```python
from build123d import *

# Parameters (mm, degrees)
SKETCH1_R           = 1.85
SKETCH1_R_2         = 4
BOSS_EXTRUDE1_DEPTH = 2


with BuildPart() as part:
    # Sketch1 → Boss-Extrude1 (new body)
    with BuildSketch(Plane.XZ):
        with BuildLine():
            Line((48, -174), (48, 14))
            ThreePointArc((48, 14), (47.414213562, 15.414213562), (46, 16))
            Line((46, 16), (-14, 16))
            ThreePointArc((-14, 16), (-15.414213562, 15.414213562), (-16, 14))
            Line((-16, 14), (-16, -174))
            ThreePointArc((-16, -174), (-15.414213562, -175.414213562), (-14, -176))
            Line((-14, -176), (46, -176))
            ThreePointArc((46, -176), (47.414213562, -175.414213562), (48, -174))
        make_face()
        with Locations((37.656854249, -154.343145751)):
            Circle(SKETCH1_R, mode=Mode.SUBTRACT)
        with Locations((26.343145751, -154.343145751)):
            Circle(SKETCH1_R, mode=Mode.SUBTRACT)
        with Locations((26.343145751, -165.656854249)):
            Circle(SKETCH1_R, mode=Mode.SUBTRACT)
        with Locations((37.656854249, -165.656854249)):
            Circle(SKETCH1_R, mode=Mode.SUBTRACT)
        with Locations((24, -160)):
            Circle(SKETCH1_R, mode=Mode.SUBTRACT)
        with Locations((32, -152)):
            Circle(SKETCH1_R, mode=Mode.SUBTRACT)
        with Locations((40, -160)):
            Circle(SKETCH1_R, mode=Mode.SUBTRACT)
        with Locations((32, -168)):
            Circle(SKETCH1_R, mode=Mode.SUBTRACT)
        with Locations((32, -160)):
            Circle(SKETCH1_R_2, mode=Mode.SUBTRACT)
        with Locations((5.656854249, -154.343145751)):
            Circle(SKETCH1_R, mode=Mode.SUBTRACT)
        with Locations((-5.656854249, -154.343145751)):
            Circle(SKETCH1_R, mode=Mode.SUBTRACT)
        with Locations((-5.656854249, -165.656854249)):
            Circle(SKETCH1_R, mode=Mode.SUBTRACT)
        with Locations((5.656854249, -165.656854249)):
            Circle(SKETCH1_R, mode=Mode.SUBTRACT)
        with Locations((-8, -160)):
            Circle(SKETCH1_R, mode=Mode.SUBTRACT)
        with Locations((0, -152)):
            Circle(SKETCH1_R, mode=Mode.SUBTRACT)
        with Locations((8, -160)):
            Circle(SKETCH1_R, mode=Mode.SUBTRACT)
        with Locations((0, -168)):
            Circle(SKETCH1_R, mode=Mode.SUBTRACT)
        with Locations((0, -160)):
            Circle(SKETCH1_R_2, mode=Mode.SUBTRACT)
        with Locations((37.656854249, -122.34314575)):
            Circle(SKETCH1_R, mode=Mode.SUBTRACT)
        with Locations((26.343145751, -122.34314575)):
            Circle(SKETCH1_R, mode=Mode.SUBTRACT)
        with Locations((26.343145751, -133.656854249)):
            Circle(SKETCH1_R, mode=Mode.SUBTRACT)
        with Locations((37.656854249, -133.656854249)):
            Circle(SKETCH1_R, mode=Mode.SUBTRACT)
        with Locations((24, -128)):
            Circle(SKETCH1_R, mode=Mode.SUBTRACT)
        with Locations((32, -120)):
            Circle(SKETCH1_R, mode=Mode.SUBTRACT)
        with Locations((40, -128)):
            Circle(SKETCH1_R, mode=Mode.SUBTRACT)
        with Locations((32, -136)):
            Circle(SKETCH1_R, mode=Mode.SUBTRACT)
        with Locations((32, -128)):
            Circle(SKETCH1_R_2, mode=Mode.SUBTRACT)
        with Locations((5.656854249, -122.34314575)):
            Circle(SKETCH1_R, mode=Mode.SUBTRACT)
        with Locations((-5.656854249, -122.34314575)):
            Circle(SKETCH1_R, mode=Mode.SUBTRACT)
        with Locations((-5.656854249, -133.656854249)):
            Circle(SKETCH1_R, mode=Mode.SUBTRACT)
        with Locations((5.656854249, -133.656854249)):
            Circle(SKETCH1_R, mode=Mode.SUBTRACT)
        with Locations((-8, -128)):
            Circle(SKETCH1_R, mode=Mode.SUBTRACT)
        with Locations((0, -120)):
            Circle(SKETCH1_R, mode=Mode.SUBTRACT)
        with Locations((8, -128)):
            Circle(SKETCH1_R, mode=Mode.SUBTRACT)
        with Locations((0, -136)):
            Circle(SKETCH1_R, mode=Mode.SUBTRACT)
        with Locations((0, -128)):
            Circle(SKETCH1_R_2, mode=Mode.SUBTRACT)
        with Locations((37.656854249, -90.343145751)):
            Circle(SKETCH1_R, mode=Mode.SUBTRACT)
        with Locations((26.343145751, -90.343145751)):
            Circle(SKETCH1_R, mode=Mode.SUBTRACT)
        with Locations((26.343145751, -101.65685425)):
            Circle(SKETCH1_R, mode=Mode.SUBTRACT)
        with Locations((37.656854249, -101.65685425)):
            Circle(SKETCH1_R, mode=Mode.SUBTRACT)
        with Locations((24, -96)):
            Circle(SKETCH1_R, mode=Mode.SUBTRACT)
        with Locations((32, -88)):
            Circle(SKETCH1_R, mode=Mode.SUBTRACT)
        with Locations((40, -96)):
            Circle(SKETCH1_R, mode=Mode.SUBTRACT)
        with Locations((32, -104)):
            Circle(SKETCH1_R, mode=Mode.SUBTRACT)
        with Locations((32, -96)):
            Circle(SKETCH1_R_2, mode=Mode.SUBTRACT)
        with Locations((5.656854249, -90.343145751)):
            Circle(SKETCH1_R, mode=Mode.SUBTRACT)
        with Locations((-5.656854249, -90.343145751)):
            Circle(SKETCH1_R, mode=Mode.SUBTRACT)
        with Locations((-5.656854249, -101.65685425)):
            Circle(SKETCH1_R, mode=Mode.SUBTRACT)
        with Locations((5.656854249, -101.65685425)):
            Circle(SKETCH1_R, mode=Mode.SUBTRACT)
        with Locations((-8, -96)):
            Circle(SKETCH1_R, mode=Mode.SUBTRACT)
        with Locations((0, -88)):
            Circle(SKETCH1_R, mode=Mode.SUBTRACT)
        with Locations((8, -96)):
            Circle(SKETCH1_R, mode=Mode.SUBTRACT)
        with Locations((0, -104)):
            Circle(SKETCH1_R, mode=Mode.SUBTRACT)
        with Locations((0, -96)):
            Circle(SKETCH1_R_2, mode=Mode.SUBTRACT)
        with Locations((37.656854249, -58.343145751)):
            Circle(SKETCH1_R, mode=Mode.SUBTRACT)
        with Locations((26.343145751, -58.343145751)):
            Circle(SKETCH1_R, mode=Mode.SUBTRACT)
        with Locations((26.343145751, -69.656854249)):
            Circle(SKETCH1_R, mode=Mode.SUBTRACT)
        with Locations((37.656854249, -69.656854249)):
            Circle(SKETCH1_R, mode=Mode.SUBTRACT)
        with Locations((24, -64)):
            Circle(SKETCH1_R, mode=Mode.SUBTRACT)
        with Locations((32, -56)):
            Circle(SKETCH1_R, mode=Mode.SUBTRACT)
        with Locations((40, -64)):
            Circle(SKETCH1_R, mode=Mode.SUBTRACT)
        with Locations((32, -72)):
            Circle(SKETCH1_R, mode=Mode.SUBTRACT)
        with Locations((32, -64)):
            Circle(SKETCH1_R_2, mode=Mode.SUBTRACT)
        with Locations((5.656854249, -58.343145751)):
            Circle(SKETCH1_R, mode=Mode.SUBTRACT)
        with Locations((-5.656854249, -58.343145751)):
            Circle(SKETCH1_R, mode=Mode.SUBTRACT)
        with Locations((-5.656854249, -69.656854249)):
            Circle(SKETCH1_R, mode=Mode.SUBTRACT)
        with Locations((5.656854249, -69.656854249)):
            Circle(SKETCH1_R, mode=Mode.SUBTRACT)
        with Locations((-8, -64)):
            Circle(SKETCH1_R, mode=Mode.SUBTRACT)
        with Locations((0, -56)):
            Circle(SKETCH1_R, mode=Mode.SUBTRACT)
        with Locations((8, -64)):
            Circle(SKETCH1_R, mode=Mode.SUBTRACT)
        with Locations((0, -72)):
            Circle(SKETCH1_R, mode=Mode.SUBTRACT)
        with Locations((0, -64)):
            Circle(SKETCH1_R_2, mode=Mode.SUBTRACT)
        Circle(SKETCH1_R_2, mode=Mode.SUBTRACT)
        with Locations((37.656854249, -26.343145751)):
            Circle(SKETCH1_R, mode=Mode.SUBTRACT)
        with Locations((26.343145751, -26.343145751)):
            Circle(SKETCH1_R, mode=Mode.SUBTRACT)
        with Locations((26.343145751, -37.656854249)):
            Circle(SKETCH1_R, mode=Mode.SUBTRACT)
        with Locations((37.656854249, -37.656854249)):
            Circle(SKETCH1_R, mode=Mode.SUBTRACT)
        with Locations((24, -32)):
            Circle(SKETCH1_R, mode=Mode.SUBTRACT)
        with Locations((32, -24)):
            Circle(SKETCH1_R, mode=Mode.SUBTRACT)
        with Locations((40, -32)):
            Circle(SKETCH1_R, mode=Mode.SUBTRACT)
        with Locations((32, -40)):
            Circle(SKETCH1_R, mode=Mode.SUBTRACT)
        with Locations((32, -32)):
            Circle(SKETCH1_R_2, mode=Mode.SUBTRACT)
        with Locations((5.656854249, -26.343145751)):
            Circle(SKETCH1_R, mode=Mode.SUBTRACT)
        with Locations((-5.656854249, -26.343145751)):
            Circle(SKETCH1_R, mode=Mode.SUBTRACT)
        with Locations((-5.656854249, -37.656854249)):
            Circle(SKETCH1_R, mode=Mode.SUBTRACT)
        with Locations((5.656854249, -37.656854249)):
            Circle(SKETCH1_R, mode=Mode.SUBTRACT)
        with Locations((-8, -32)):
            Circle(SKETCH1_R, mode=Mode.SUBTRACT)
        with Locations((0, -24)):
            Circle(SKETCH1_R, mode=Mode.SUBTRACT)
        with Locations((8, -32)):
            Circle(SKETCH1_R, mode=Mode.SUBTRACT)
        with Locations((0, -40)):
            Circle(SKETCH1_R, mode=Mode.SUBTRACT)
        with Locations((0, -32)):
            Circle(SKETCH1_R_2, mode=Mode.SUBTRACT)
        with Locations((37.656854249, 5.656854249)):
            Circle(SKETCH1_R, mode=Mode.SUBTRACT)
        with Locations((26.343145751, 5.656854249)):
            Circle(SKETCH1_R, mode=Mode.SUBTRACT)
        with Locations((26.343145751, -5.656854249)):
            Circle(SKETCH1_R, mode=Mode.SUBTRACT)
        with Locations((37.656854249, -5.656854249)):
            Circle(SKETCH1_R, mode=Mode.SUBTRACT)
        with Locations((24, 0)):
            Circle(SKETCH1_R, mode=Mode.SUBTRACT)
        with Locations((32, 8)):
            Circle(SKETCH1_R, mode=Mode.SUBTRACT)
        with Locations((40, 0)):
            Circle(SKETCH1_R, mode=Mode.SUBTRACT)
        with Locations((32, -8)):
            Circle(SKETCH1_R, mode=Mode.SUBTRACT)
        with Locations((32, 0)):
            Circle(SKETCH1_R_2, mode=Mode.SUBTRACT)
        with Locations((5.656854249, 5.656854249)):
            Circle(SKETCH1_R, mode=Mode.SUBTRACT)
        with Locations((-5.656854249, 5.656854249)):
            Circle(SKETCH1_R, mode=Mode.SUBTRACT)
        with Locations((-5.656854249, -5.656854249)):
            Circle(SKETCH1_R, mode=Mode.SUBTRACT)
        with Locations((5.656854249, -5.656854249)):
            Circle(SKETCH1_R, mode=Mode.SUBTRACT)
        with Locations((-8, 0)):
            Circle(SKETCH1_R, mode=Mode.SUBTRACT)
        with Locations((0, 8)):
            Circle(SKETCH1_R, mode=Mode.SUBTRACT)
        with Locations((8, 0)):
            Circle(SKETCH1_R, mode=Mode.SUBTRACT)
        with Locations((0, -8)):
            Circle(SKETCH1_R, mode=Mode.SUBTRACT)
    extrude(amount=-BOSS_EXTRUDE1_DEPTH)


solid = part.part
```
Verification items for the finished model (mm, model axes). Round coordinates to 2 decimals unless told otherwise and drop trailing zeros. Write each loop counter-clockwise with the first axis right and the second up, starting at its lowest first coordinate (ties: lowest second). Pieces come first, ordered by that corner, then holes. Notation, with made-up numbers: (-10, 15) - (27, 15) arc R25 cw to (27, 43) - close; hole circle Ø4 at (-38.5, 57.5). An arc over 180 degrees is marked (long way). Answer as a JSON object with one key per item and string values. Group by question number.
Q1. Go/stop test with flat-tipped pins: pin 1 Ø5 at (x, z) = (24, -32) entering from -Y; pin 2 Ø2 at (x, z) = (37.66, -90.34) entering from +Y. Record where each tip stops, or that it passes through.
Q2. Thickness scan on line 1 (X direction, y = 0.55, z = -104); line 2 (X direction, y = 1.5, z = -37); line 3 (X direction, y = 1.75, z = -23). Record the ranges inside material, lowest first.
Q3. Section check B-B, the plane x = 0. Give the number of separate pieces and of enclosed holes in the cut face, plus the area to 3 significant figures.
Q4. Section check A-A, the plane z = -64. Enter the section's corners in (x, y).
Found:
{
 "1": {"pin 1": "stops at y = 0", "pin 2": "passes through"},
 "2": {"line 1": "x = -16 to -1.85, 1.85 to 30.15, 33.85 to 48", "line 2": "x = -16 to -7.39, -3.93 to 3.93, 7.39 to 24.61, 28.07 to 35.93, 39.39 to 48", "line 3": "x = -16 to -1.56, 1.56 to 30.44, 33.56 to 48"},
 "3": {"separate pieces": "19", "enclosed holes": "0", "area": "199 mm^2"},
 "4": {"outline": "(-16, 0) - (-9.85, 0) - (-9.85, 2) - (-16, 2) - close; (-6.15, 0) - (-4, 0) - (-4, 2) - (-6.15, 2) - close; (4, 0) - (6.15, 0) - (6.15, 2) - (4, 2) - close; (9.85, 0) - (22.15, 0) - (22.15, 2) - (9.85, 2) - close; (25.85, 0) - (28, 0) - (28, 2) - (25.85, 2) - close; (36, 0) - (38.15, 0) - (38.15, 2) - (36, 2) - close; (41.85, 0) - (48, 0) - (48, 2) - (41.85, 2) - close"}
}
